Model file for the job. Use its own axes, mm. Face numbers are marked on the shaded views. A direction names the side the tool comes from. Give positions to 0.01 mm unless a question says otherwise; leave off trailing zeros. Order: outer loops, then holes, each group sorted by start corner. A loop starts at its lowest first (then second) coordinate and runs counter-clockwise, first axis right, second up. Notation, with made-up numbers: (89.25, 29) -> (147.25, 29) arc R21 cw to (147.25, 60) -> close; hole circle Ø2 at (9.5, 64.5). An arc over 180 degrees is marked (long way). Answer in a Markdown table with one row per item. Add a question column.
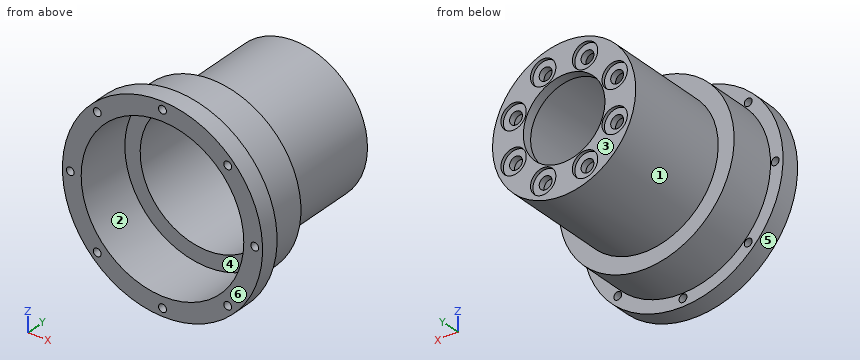
from build123d import *

# Parameters (mm, degrees)
HOLE_WIZARD_M3_1_D       = 2.5
PATTERN_CIRCULAR_1_COUNT = 2
PATTERN_CIRCULAR_1_ANGLE = 45
SKETCH_5_R               = 2.05
CUT_EXTRUDE_1_DEPTH      = 10
PATTERN_CIRCULAR_2_COUNT = 8
SKETCH_6_R               = 4.05
CUT_EXTRUDE_2_DEPTH      = 1
PATTERN_CIRCULAR_3_COUNT = 8


with BuildPart() as part:
    # 草图1 → 旋转1 (revolve)
    with BuildSketch(Plane.XY, mode=Mode.PRIVATE) as revolve_1_sk:
        Polygon((32, 0), (32, 6), (28, 6), (28, 21), (22.9, 21), (22.9, 55), (13.05, 55), (13.05, 52), (21.1, 52), (21.1, 18), (26, 18), (26, 0), align=None)
    revolve(revolve_1_sk.sketch.rotate(Axis((0, 0, 0), (0, 1, 0)), 90), axis=Axis((0, 0, 0), (0, 1, 0)))

    # M3 螺纹孔1 (through all)
    with Locations(Plane(origin=(0, 0, 0), x_dir=(-1, 0, 0), z_dir=(0, -1, 0))):
        with Locations((0, 29.5), (29.5, 0), (0, -29.5), (-29.5, 0)):
            hole_wizard_m3_1 = Hole(HOLE_WIZARD_M3_1_D / 2)

    # 阵列(圆周)1: M3 螺纹孔1 ×2 about axis
    pattern_circular_1_axis = Axis((0, 0, 0), (0, -1, 0))
    for i in range(1, PATTERN_CIRCULAR_1_COUNT):
        add(hole_wizard_m3_1.rotate(pattern_circular_1_axis, i * PATTERN_CIRCULAR_1_ANGLE / (PATTERN_CIRCULAR_1_COUNT - 1)), mode=Mode.SUBTRACT)

    # 草图5 → 切除-拉伸1 (cut)
    with BuildSketch(Plane(origin=(0, 55, 0), x_dir=(1, 0, 0), z_dir=(0, 1, 0))):
        with Locations(Location((-6.696960066, 16.167891819, 0), (0, 0, 270))):
            Circle(SKETCH_5_R)
    cut_extrude_1 = extrude(amount=-CUT_EXTRUDE_1_DEPTH, mode=Mode.SUBTRACT)

    # 阵列(圆周)2: 切除-拉伸1 ×8 about axis
    pattern_circular_2_axis = Axis((0, 0, 0), (0, 1, 0))
    for i in range(1, PATTERN_CIRCULAR_2_COUNT):
        add(cut_extrude_1.rotate(pattern_circular_2_axis, i * 360 / PATTERN_CIRCULAR_2_COUNT), mode=Mode.SUBTRACT)

    # 草图6 → 切除-拉伸2 (cut)
    with BuildSketch(Plane(origin=(0, 55, 0), x_dir=(1, 0, 0), z_dir=(0, 1, 0))):
        with Locations(Location((-6.696960066, 16.167891819, 0), (0, 0, 270))):
            Circle(SKETCH_6_R)
    cut_extrude_2 = extrude(amount=-CUT_EXTRUDE_2_DEPTH, mode=Mode.SUBTRACT)

    # 阵列(圆周)3: 切除-拉伸2 ×8 about axis
    pattern_circular_3_axis = Axis((0, 0, 0), (0, 1, 0))
    for i in range(1, PATTERN_CIRCULAR_3_COUNT):
        add(cut_extrude_2.rotate(pattern_circular_3_axis, i * 360 / PATTERN_CIRCULAR_3_COUNT), mode=Mode.SUBTRACT)


solid = part.part
Item 1: Saw through at C-C on y = 47.5. List the corners of the cut face in (x, z), plus the area to 3 significant figures.
Item 2: Which spindle directions (+Z, -Z, +X, -X, +Y, -Y) get a long thin tool onto all of the face, cutting with end or side? Do the marked faces 1, 2 and 3. Say none if no direction does.
Item 3: Wall check: line 1 (Z direction, x = 13, y = 14); line 2 (X direction, y = 32.5, z = -11); line 3 (X direction, y = 37, z = 5). Give the ranges that are in metal, low to high.
Item 4: Saw through at A-A on z = 0. Give the number of separate pieces and of enclosed holes in the cut face, plus the area to 3 significant figures.
Item 5: Two-plate mould, pull along Z, no slides. Class the marked faces 4, 5 and 6: pulls with the +Z half, pulls with the -Z half, needs draft (parallel to the pull), parting line crosses it, or undercut.
Item 6: Pin check, flat tips, straight feed: pin 1 Ø5 at (x, y) = (-7.5, 15.5) entering from +Z; pin 2 Ø2.5 at (x, z) = (14, -6) entering from +Y; pin 3 Ø1 at (x, y) = (16.5, 33.5) entering from -Z. Stop position of each tip, or through.
Item 7: Saw through at D-D on x = -29.5. List the corners of the cut face in (y, z).
Evaluation:
| question | item | result |
|---|---|---|
| 1 | outline | circle Ø45.8 at (0, 0); hole circle Ø42.2 at (0, 0) |
| 1 | area | 249 mm2 |
| 2 | face 1 | +Y |
| 2 | face 2 | -Y |
| 2 | face 3 | +Z, -Z, +X, -X, +Y |
| 3 | line 1 | z = -24.8 to -22.52, 22.52 to 24.8 |
| 3 | line 2 | x = -20.09 to -18.01, 18.01 to 20.09 |
| 3 | line 3 | x = -22.35 to -20.5, 20.5 to 22.35 |
| 4 | separate pieces | 4 |
| 4 | enclosed holes | 0 |
| 4 | area | 302 mm2 |
| 5 | face 4 | undercut |
| 5 | face 5 | parting line crosses it |
| 5 | face 6 | needs draft |
| 6 | pin 1 | stops at z = 27.55 |
| 6 | pin 2 | stops at y = 54 |
| 6 | pin 3 | stops at z = -16.38 |
| 7 | outline | (0, -12.4) -> (6, -12.4) -> (6, -1.25) -> (0, -1.25) -> close; (0, 1.25) -> (6, 1.25) -> (6, 12.4) -> (0, 12.4) -> close |
